Design review of the part built by this model. Coordinates are the model's own, in mm. A direction names the side the tool comes from. Coordinates: 2 decimals unless noted, no trailing zeros. Loops run counter-clockwise (first coordinate to the right, second up) from the corner with the lowest first, then second, coordinate; pieces in that order, holes last. Notation, with made-up numbers: M 89.5,83 L 108.5,83 A26 cw 108.5,122 Z; hole C 78.25,89.5 d10. An arc over 180 degrees is marked long. Write item = value, one per line. Start each with the question number.
```python
from build123d import *

# Parameters (mm, degrees)
SKETCH1_W           = 30.8
SKETCH1_H           = 13
SKETCH1_R           = 1.89865
BOSS_EXTRUDE1_DEPTH = 3.175
FILLET1_R           = 0.5


with BuildPart() as part:
    # Sketch1 → Boss-Extrude1 (new body)
    with BuildSketch(Plane(origin=(0, 0, 0), x_dir=(1, 0, 0), z_dir=(0, 1, 0))):
        with Locations((15.4, 6.5)):
            Rectangle(SKETCH1_W, SKETCH1_H)
        with Locations(Location((7.5, 6.5, 0), (0, 0, 270))):
            Circle(SKETCH1_R, mode=Mode.SUBTRACT)
        Polygon((27.8, 5.229289322), (27.8, 7.770710678), (26.120710678, 9.45), (17.5, 9.45), (17.5, 3.55), (26.120710678, 3.55), align=None, mode=Mode.SUBTRACT)
    extrude(amount=BOSS_EXTRUDE1_DEPTH)

    # Fillet1
    fillet1_edges = [part.edges().sort_by_distance(p)[0] for p in [
        (0, 1.5875, -13),
        (30.8, 1.5875, -13),
        (30.8, 1.5875, 0),
        (0, 1.5875, 0),
    ]]
    fillet(fillet1_edges, radius=FILLET1_R)


solid = part.part
```
(1) Mouldability with a two-part tool opening along X and no side actions: class faces 3 (the flat face through (15, 2, -13)), 4 (the flat face through (0, 2, -6)), 5 (the flat face through (17.5, 2, -7)) as +X half, -X half, draft (parallel to the pull), parting line (faces both ways), or undercut.
(2) Take a section at B-B (y = 2.75). State the section outline as (x, z) points.
(3) To check wall thickness, follow L1, parallel to X at y = 2.55, z = -6.5; L2, parallel to X at y = 2.35, z = -5.5; L3, parallel to Z at x = 25, y = 1.2. State the ranges of each line that lie inside material, in increasing order.
(4) Insertion check: pin 1 (1 mm diameter, centred on x = 10.5, z = -4, fed in from -Y). The pin has a flat end and moves straight along its axis. Give the tip position at first contact, or say it passes through.
(5) Take a section at D-D (z = -8.75). State the section outline as (x, y) points (3 decimals), plus the area to 3 significant figures.
(6) Take a section at C-C (z = -6.5). State the section outline as (x, y) points (3 decimals), plus the area to 3 significant figures.
(7) Take a section at A-A (x = 7.5). State the section outline as (y, z) points (3 decimals), plus the area to 3 significant figures.
(8) Tool access review of faces 1 (the flat face through (22, 2, -3.55)), 2 (the flat face through (15, 0, -7)): name each direction out of +Z, -Z, +X, -X, +Y, -Y from which nothing blocks a thin tool from reaching the whole face with its end or side.
Results list:
q1.face_3 = draft
q1.face_4 = -X half
q1.face_5 = undercut
q2.outline = M 0,-12.5 A0.5 ccw 0.5,-13 L 30.3,-13 A0.5 ccw 30.8,-12.5 L 30.8,-0.5 A0.5 ccw 30.3,0 L 0.5,0 A0.5 ccw 0,-0.5 Z; hole C 7.5,-6.5 d3.8; hole M 17.5,-9.45 L 26.12,-9.45 L 27.8,-7.77 L 27.8,-5.23 L 26.12,-3.55 L 17.5,-3.55 Z
q3.L1 = 0 to 5.6, 9.4 to 17.5, 27.8 to 30.8
q3.L2 = 0 to 5.89, 9.11 to 17.5, 27.8 to 30.8
q3.L3 = -13 to -9.45, -3.55 to 0
q4.pin_1 = 0
q5.outline = M 0,0 L 17.5,0 L 17.5,3.175 L 0,3.175 Z; M 26.821,0 L 30.8,0 L 30.8,3.175 L 26.821,3.175 Z
q5.area = 68.2 mm^2
q6.outline = M 0,0 L 5.601,0 L 5.601,3.175 L 0,3.175 Z; M 9.399,0 L 17.5,0 L 17.5,3.175 L 9.399,3.175 Z; M 27.8,0 L 30.8,0 L 30.8,3.175 L 27.8,3.175 Z
q6.area = 53.0 mm^2
q7.outline = M 0,-13 L 3.175,-13 L 3.175,-8.399 L 0,-8.399 Z; M 0,-4.601 L 3.175,-4.601 L 3.175,0 L 0,0 Z
q7.area = 29.2 mm^2
q8.face_1 = +Y, -Y
q8.face_2 = +Z, -Z, +X, -X, -Y
